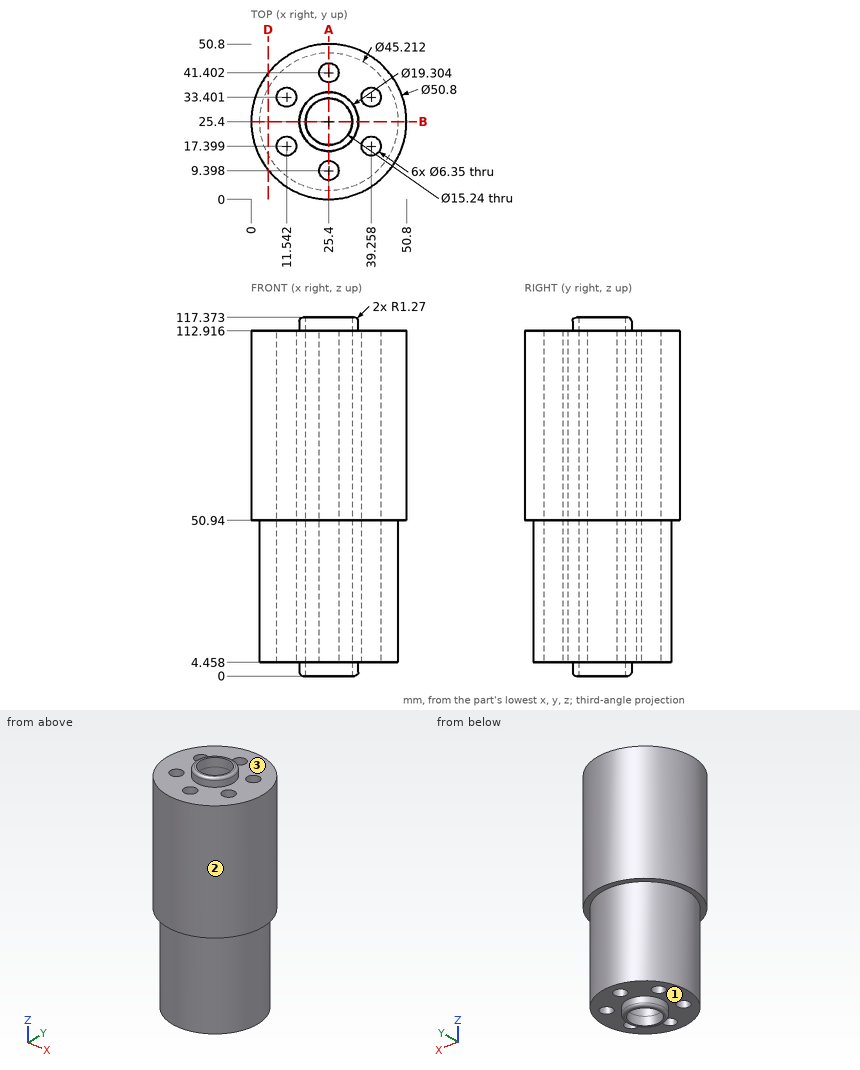
Part print with two shaded views. Sizes in mm from the minimum x, y, z corner. A direction names the side the tool comes from. Coordinates: 2 decimals unless noted, no trailing zeros. Write each loop counter-clockwise with the first axis right and the second up, starting at its lowest first coordinate (ties: lowest second). Pieces come first, ordered by that corner, then holes. Notation, with made-up numbers: M 78.5,-1 L 113.5,-1 A21 ccw 113.5,3 Z; hole C 74.5,59.25 d11. An arc over 180 degrees is marked long. Return JSON: item names as keys, results as strings.
Item 1: Probe line 1 (Y direction, x = 25, z = 84); line 2 (X direction, y = 25, z = 2); line 3 (X direction, y = 19.5, z = 91.5) (1 decimal). List the from-to ranges inside material, lowest first. Write a range as from..to.
Findings below:
{"line 1": "y = 0..6.25, 12.55..17.79, 33.01..38.25, 44.55..50.8", "line 2": "x = 15.76..17.79, 33.01..35.04", "line 3": "x = 0.7..9.2, 13.9..20.6, 30.2..36.9, 41.6..50.1"}
Item 2: Slice it at D-D, the plane x = 5.5. Write the cut outline in (y, z) (1 decimal).
Findings below:
{"outline": "M 9.6,50.9 L 14.7,50.9 L 14.7,4.5 L 36.1,4.5 L 36.1,50.9 L 41.2,50.9 L 41.2,112.9 L 9.6,112.9 Z"}
Item 3: Drop flat-ended pins along their axis: pin 1 Ø8.5 at (x, y) = (39.26, 17.4) entering from +Z; pin 2 Ø6 at (y, z) = (42.5, 74) entering from +X; pin 3 Ø1 at (y, z) = (9, 99.5) entering from +X. Give the stop position or say it passes through.
Findings below:
{"pin 1": "stops at z = 112.92", "pin 2": "stops at x = 46.53", "pin 3": "stops at x = 45.21"}
Item 4: Slice it at A-A, the plane x = 25.4. State how many separate pieces and enclosed holes the cut face has.
Findings below:
{"separate pieces": "4", "enclosed holes": "0"}
Item 5: Which spindle directions (+Z, -Z, +X, -X, +Y, -Y) get a long thin tool onto all of the face, cutting with end or side? Do the marked faces 1, 2 and 3. Say none if no direction does.
Findings below:
{"face 1": "-Z", "face 2": "+Z, -Z", "face 3": "+Z"}
Item 6: Slice it at B-B, the plane y = 25.4. Write the cut outline in (x, z) (1 decimal), and give its area (3 significant figures).
Findings below:
{"outline": "M 0,50.9 L 2.8,50.9 L 2.8,4.5 L 15.7,4.5 L 15.7,1.3 A1.3 ccw 17,0 L 17.8,0 L 17.8,117.4 L 17,117.4 A1.3 ccw 15.7,116.1 L 15.7,112.9 L 0,112.9 Z; M 33,0 L 33.8,0 A1.3 ccw 35.1,1.3 L 35.1,4.5 L 48,4.5 L 48,50.9 L 50.8,50.9 L 50.8,112.9 L 35.1,112.9 L 35.1,116.1 A1.3 ccw 33.8,117.4 L 33,117.4 Z", "area": "3,630 mm2"}
